Can you work these out from the drawing? Everything is in mm from the part's minimum corner. A direction names the side the tool comes from. Coordinates: 2 decimals unless noted, no trailing zeros. Write each loop counter-clockwise with the first axis right and the second up, starting at its lowest first coordinate (ties: lowest second). Pieces come first, ordered by that corner, then holes. Notation, with made-up numbers: M 21.25,86 L 71.25,86 A28 cw 71.25,122 Z; hole C 37,-36.75 d11. An arc over 180 degrees is marked long. Write item = value, one per line.
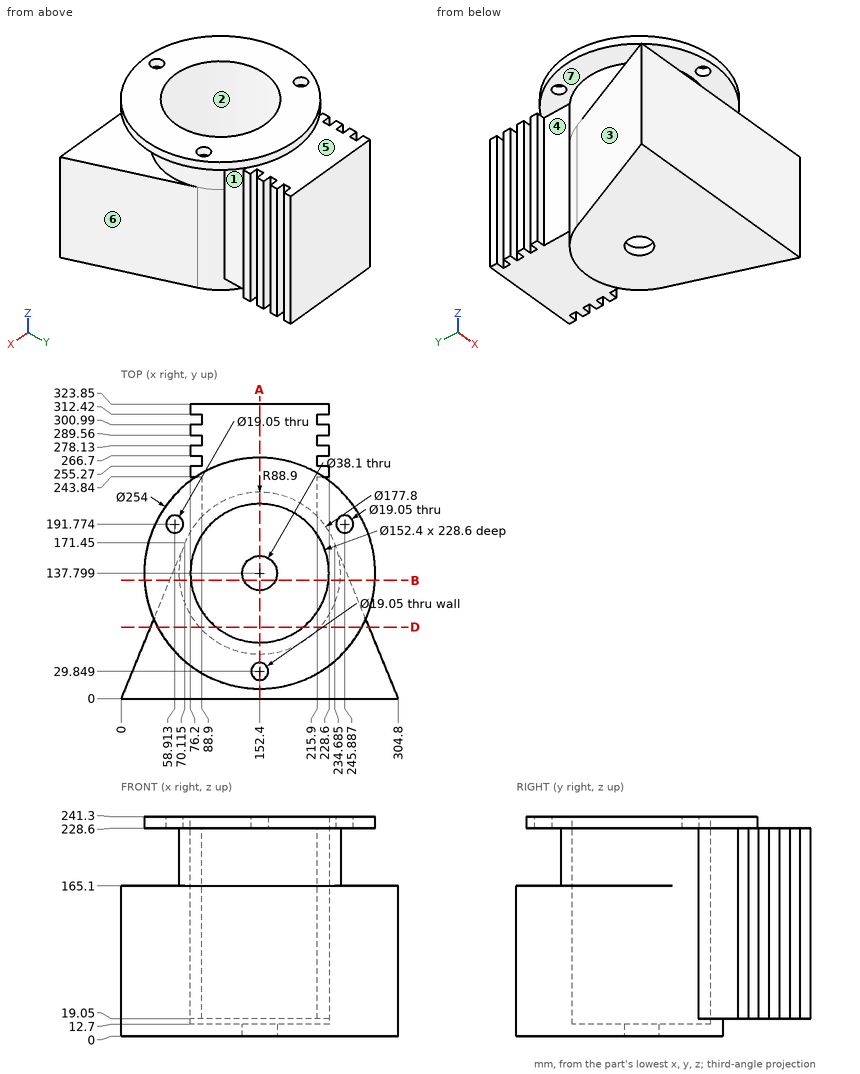
Item 1: If I drill on line 1 along Z through (x, y) = (90.5, 45); line 2 along Y through (x, z) = (152.4, 173); line 3 along Y through (x, z) = (152, 87), over which ranges is the centre line in solid material (lowest first)?
Numbers:
line_1 = 0 to 165.1, 228.6 to 241.3
line_2 = 48.9 to 61.6, 214 to 323.85
line_3 = 0 to 61.6, 214 to 323.85
Item 2: Imagine slicing it at A-A (x = 152.4). State how many separate pieces and enclosed holes the cut face has, and give its area (3 significant figures).
Numbers:
separate_pieces = 3
enclosed_holes = 0
area = 36,700 mm²
Item 3: Imagine slicing it at D-D (y = 78.5). Write out the boundary of the cut face in (x, z) (1 decimal).
Numbers:
outline = M 32.1,0 L 272.7,0 L 272.7,165.1 L 218.6,165.1 L 218.6,228.6 L 264.7,228.6 L 264.7,241.3 L 200.3,241.3 L 200.3,12.7 L 104.5,12.7 L 104.5,241.3 L 40.1,241.3 L 40.1,228.6 L 86.2,228.6 L 86.2,165.1 L 32.1,165.1 Z
Item 4: I'm going to push flat-ended pins straight in: P1, Ø1, axis at x = 183.5, y = 40.5, coming from the -Z side; P2, Ø1.5, axis at y = 225, z = 92, coming from the +X side; P3, Ø3.5, axis at y = 249.5, z = 83.5, coming from the -X side; P4, Ø4, axis at x = 76, z = 209, coming from the -Y side. Where does each tip first touch, or does it pass through?
Numbers:
P1 = 0
P2 = 215.9
P3 = 76.2
P4 = 89.14
Item 5: For the marked faces 1, 2, 3 and 4, which set-ups out of +Z, -Z, +X, -X, +Y, -Y let a thin tool reach every point of the face, with its end or its side?
Numbers:
face_1 = -Z, +X
face_2 = +Z
face_3 = -Z, -X, +Y
face_4 = -Z, -X
Item 6: If we mould it in two halves opening along Z, with no side actions, what happens to the marked faces 5, 6 and 7? For each: pulls with the +Z half, pulls with the -Z half, needs draft (parallel to the pull), parting line crosses it, or undercut.
Numbers:
face_5 = pulls with the +Z half
face_6 = needs draft
face_7 = undercut
Item 7: Imagine slicing it at B-B (y = 130). Write out the boundary of the cut face in (x, z).
Numbers:
outline = M 25.64,228.6 L 63.84,228.6 L 63.84,165.1 L 53.16,165.1 L 53.16,0 L 135.02,0 L 135.02,12.7 L 76.6,12.7 L 76.6,241.3 L 25.64,241.3 Z; M 169.78,0 L 251.64,0 L 251.64,165.1 L 240.96,165.1 L 240.96,228.6 L 279.16,228.6 L 279.16,241.3 L 228.2,241.3 L 228.2,12.7 L 169.78,12.7 Z
